For this review, take the finished solid that the model builds, in its own axes (mm). A direction names the side the tool comes from. Give positions to 0.01 mm unless a question says otherwise; leave off trailing zeros. Write each loop counter-clockwise with the first axis right and the second up, starting at its lowest first coordinate (ties: lowest second). Pieces come first, ordered by that corner, then holes.
1) For P1, Ø1.5, axis at y = 68, z = 1.5, coming from the -X side; P2, Ø1.5, axis at y = 65.5, z = 1.5, coming from the +X side; P3, Ø1.9, axis at x = 55.87, y = -64.6, coming from the +Z side; P4, Ø1, axis at x = -56.5, z = 1, coming from the +Y side, all flat-tipped, find the tip position at first contact; note any pin that passes through.
2) Wall thickness on line 1 along X through (y, z) = (19, 0.45); line 2 along Y through (x, z) = (-2.5, 1.2); line 3 along X through (y, z) = (44, 0.6): over which ranges is each line inside the solid? List them lowest first.
3) We need section C-C on z = 1.75. Give the number of separate pieces and of enclosed holes in the cut face, and give its area (3 significant figures).
4) Machinability: for faces 5 (the face through (68.796, -68.889, 1.479)), 6 (the face through (-51.49, 51.72, 1.48)), which of the approach directions +Z, -Z, +X, -X, +Y, -Y give a long, thin tool a straight path to every point of the face, cutting with its end or side? Answer none if there is none.
5) Draft analysis for pull direction Y (two halves, no side actions). For faces 1 (the face through (25.348, 85.358, 1.479)), 2 (the face through (38.828, 81.603, 1.479)), 3 (the face through (-68.889, -68.796, 1.479)), 4 (the face through (50.091, 50.293, 1.479)), state which applies: pulls with the +Y half, pulls with the -Y half, needs draft (parallel to the pull), parting line crosses it, or undercut.
6) We need section B-B on y = 9.5. Give the boundary of the cut face in (x, z).
7) We need section A-A on x = -5. Give the boundary of the cut face in (y, z).
from build123d import *

# Parameters (mm, degrees)
SKETCH2_R           = 1.6
SKETCH2_R_2         = 2.5
SKETCH2_W           = 82
SKETCH2_H           = 12.6
BOSS_EXTRUDE1_DEPTH = 3
FILLET2_R           = 1.5
FILLET3_R           = 3


with BuildPart() as part:
    # Sketch2 → Boss-Extrude1 (new body)
    # profile 1 of 2: a face of its own
    with BuildSketch(Plane.XY):
        with BuildLine():
            ThreePointArc((-65.540902989, 70.525765905), (-69.163190657, 68.495804286), (-70.6, 64.6))
            Line((-70.6, 64.6), (-70.6, -64.6))
            ThreePointArc((-70.6, -64.6), (-68.842640687, -68.842640687), (-64.6, -70.6))
            Line((-64.6, -70.6), (64.6, -70.6))
            ThreePointArc((64.6, -70.6), (68.842640687, -68.842640687), (70.6, -64.6))
            Line((70.6, -64.6), (70.6, 64.6))
            ThreePointArc((70.6, 64.6), (69.163190657, 68.495804286), (65.540902989, 70.525765905))
            ThreePointArc((65.540902989, 70.525765905), (64.340790015, 70.792848887), (63.182522555, 71.205184867))
            Line((63.182522555, 71.205184867), (13.781138102, 92.296857547))
            ThreePointArc((13.781138102, 92.296857547), (11.858510235, 92.897157125), (9.854586018, 93.1))
            Line((9.854586018, 93.1), (-9.854586018, 93.1))
            ThreePointArc((-9.854586018, 93.1), (-11.858510235, 92.897157125), (-13.781138102, 92.296857547))
            Line((-13.781138102, 92.296857547), (-63.182522555, 71.205184867))
            ThreePointArc((-63.182522555, 71.205184867), (-64.340790015, 70.792848887), (-65.540902989, 70.525765905))
        make_face()
        with Locations((-55.87, -64.6)):
            Circle(SKETCH2_R, mode=Mode.SUBTRACT)
        with Locations((-48.6, -64.6)):
            Circle(SKETCH2_R_2, mode=Mode.SUBTRACT)
        with BuildLine():
            Line((-11.9, 91.1), (-6, 91.1))
            Line((-6, 91.1), (6, 91.1))
            Line((6, 91.1), (11.9, 91.1))
            Line((11.9, 91.1), (41, 78.675901328))
            Line((41, 78.675901328), (41, 56))
            Line((41, 56), (-41, 56))
            ThreePointArc((-41, 56), (-51.606601718, 51.606601718), (-56, 41))
            Line((-56, 41), (-56, -41))
            ThreePointArc((-56, -41), (-55.457696912, -44.996873778), (-53.87, -48.704745291))
            Line((-53.87, -48.704745291), (-53.87, -61.6))
            Line((-53.87, -61.6), (-58.87, -61.6))
            Line((-58.87, -61.6), (-58.87, -68.6))
            Line((-58.87, -68.6), (-64.6, -68.6))
            ThreePointArc((-64.6, -68.6), (-67.428427125, -67.428427125), (-68.6, -64.6))
            Line((-68.6, -64.6), (-68.6, 64.6))
            ThreePointArc((-68.6, 64.6), (-67.428427125, 67.428427125), (-64.6, 68.6))
            Line((-64.6, 68.6), (-11.9, 91.1))
        make_face(mode=Mode.SUBTRACT)
        with Locations((0, -62.3)):
            Rectangle(SKETCH2_W, SKETCH2_H, mode=Mode.SUBTRACT)
        with Locations((48.6, -64.6)):
            Circle(SKETCH2_R_2, mode=Mode.SUBTRACT)
        with Locations((55.87, -64.6)):
            Circle(SKETCH2_R, mode=Mode.SUBTRACT)
        with BuildLine():
            Line((41, -54), (-41, -54))
            ThreePointArc((-41, -54), (-50.192388155, -50.192388155), (-54, -41))
            Line((-54, -41), (-54, 41))
            ThreePointArc((-54, 41), (-50.192388155, 50.192388155), (-41, 54))
            Line((-41, 54), (41, 54))
            ThreePointArc((41, 54), (50.192388155, 50.192388155), (54, 41))
            Line((54, 41), (54, -41))
            ThreePointArc((54, -41), (50.192388155, -50.192388155), (41, -54))
        make_face(mode=Mode.SUBTRACT)
        with BuildLine():
            Line((58.972044185, 61.502827435), (58.972044185, 71.002827435))
            Line((58.972044185, 71.002827435), (64.6, 68.6))
            ThreePointArc((64.6, 68.6), (67.428427125, 67.428427125), (68.6, 64.6))
            Line((68.6, 64.6), (68.6, -64.6))
            ThreePointArc((68.6, -64.6), (67.428427125, -67.428427125), (64.6, -68.6))
            Line((64.6, -68.6), (58.87, -68.6))
            Line((58.87, -68.6), (58.87, -61.6))
            Line((58.87, -61.6), (53.87, -61.6))
            Line((53.87, -61.6), (53.87, -48.704745291))
            ThreePointArc((53.87, -48.704745291), (55.457696912, -44.996873778), (56, -41))
            Line((56, -41), (56, 41))
            ThreePointArc((56, 41), (55.354105036, 45.354270159), (53.472044185, 49.333553495))
            Line((53.472044185, 49.333553495), (53.472044185, 61.502827435))
            Line((53.472044185, 61.502827435), (58.972044185, 61.502827435))
        make_face(mode=Mode.SUBTRACT)
        with Locations((48.6, 64.6)):
            Circle(SKETCH2_R_2, mode=Mode.SUBTRACT)
        with Locations((55.87, 64.6)):
            Circle(SKETCH2_R, mode=Mode.SUBTRACT)
    # profile 2 of 2: a face of its own
    with BuildSketch(Plane.XY):
        with BuildLine():
            ThreePointArc((-65.540902989, 70.525765905), (-69.163190657, 68.495804286), (-70.6, 64.6))
            Line((-70.6, 64.6), (-70.6, -64.6))
            ThreePointArc((-70.6, -64.6), (-68.842640687, -68.842640687), (-64.6, -70.6))
            Line((-64.6, -70.6), (64.6, -70.6))
            ThreePointArc((64.6, -70.6), (68.842640687, -68.842640687), (70.6, -64.6))
            Line((70.6, -64.6), (70.6, 64.6))
            ThreePointArc((70.6, 64.6), (69.163190657, 68.495804286), (65.540902989, 70.525765905))
            ThreePointArc((65.540902989, 70.525765905), (64.340790015, 70.792848887), (63.182522555, 71.205184867))
            Line((63.182522555, 71.205184867), (13.781138102, 92.296857547))
            ThreePointArc((13.781138102, 92.296857547), (11.858510235, 92.897157125), (9.854586018, 93.1))
            Line((9.854586018, 93.1), (-9.854586018, 93.1))
            ThreePointArc((-9.854586018, 93.1), (-11.858510235, 92.897157125), (-13.781138102, 92.296857547))
            Line((-13.781138102, 92.296857547), (-63.182522555, 71.205184867))
            ThreePointArc((-63.182522555, 71.205184867), (-64.340790015, 70.792848887), (-65.540902989, 70.525765905))
        make_face()
        with Locations((-55.87, -64.6)):
            Circle(SKETCH2_R, mode=Mode.SUBTRACT)
        with Locations((-48.6, -64.6)):
            Circle(SKETCH2_R_2, mode=Mode.SUBTRACT)
        with BuildLine():
            Line((-11.9, 91.1), (-6, 91.1))
            Line((-6, 91.1), (6, 91.1))
            Line((6, 91.1), (11.9, 91.1))
            Line((11.9, 91.1), (41, 78.675901328))
            Line((41, 78.675901328), (41, 56))
            Line((41, 56), (-41, 56))
            ThreePointArc((-41, 56), (-51.606601718, 51.606601718), (-56, 41))
            Line((-56, 41), (-56, -41))
            ThreePointArc((-56, -41), (-55.457696912, -44.996873778), (-53.87, -48.704745291))
            Line((-53.87, -48.704745291), (-53.87, -61.6))
            Line((-53.87, -61.6), (-58.87, -61.6))
            Line((-58.87, -61.6), (-58.87, -68.6))
            Line((-58.87, -68.6), (-64.6, -68.6))
            ThreePointArc((-64.6, -68.6), (-67.428427125, -67.428427125), (-68.6, -64.6))
            Line((-68.6, -64.6), (-68.6, 64.6))
            ThreePointArc((-68.6, 64.6), (-67.428427125, 67.428427125), (-64.6, 68.6))
            Line((-64.6, 68.6), (-11.9, 91.1))
        make_face(mode=Mode.SUBTRACT)
        with Locations((0, -62.3)):
            Rectangle(SKETCH2_W, SKETCH2_H, mode=Mode.SUBTRACT)
        with Locations((48.6, -64.6)):
            Circle(SKETCH2_R_2, mode=Mode.SUBTRACT)
        with Locations((55.87, -64.6)):
            Circle(SKETCH2_R, mode=Mode.SUBTRACT)
        with BuildLine():
            Line((41, -54), (-41, -54))
            ThreePointArc((-41, -54), (-50.192388155, -50.192388155), (-54, -41))
            Line((-54, -41), (-54, 41))
            ThreePointArc((-54, 41), (-50.192388155, 50.192388155), (-41, 54))
            Line((-41, 54), (41, 54))
            ThreePointArc((41, 54), (50.192388155, 50.192388155), (54, 41))
            Line((54, 41), (54, -41))
            ThreePointArc((54, -41), (50.192388155, -50.192388155), (41, -54))
        make_face(mode=Mode.SUBTRACT)
        with BuildLine():
            Line((58.972044185, 61.502827435), (58.972044185, 71.002827435))
            Line((58.972044185, 71.002827435), (64.6, 68.6))
            ThreePointArc((64.6, 68.6), (67.428427125, 67.428427125), (68.6, 64.6))
            Line((68.6, 64.6), (68.6, -64.6))
            ThreePointArc((68.6, -64.6), (67.428427125, -67.428427125), (64.6, -68.6))
            Line((64.6, -68.6), (58.87, -68.6))
            Line((58.87, -68.6), (58.87, -61.6))
            Line((58.87, -61.6), (53.87, -61.6))
            Line((53.87, -61.6), (53.87, -48.704745291))
            ThreePointArc((53.87, -48.704745291), (55.457696912, -44.996873778), (56, -41))
            Line((56, -41), (56, 41))
            ThreePointArc((56, 41), (55.354105036, 45.354270159), (53.472044185, 49.333553495))
            Line((53.472044185, 49.333553495), (53.472044185, 61.502827435))
            Line((53.472044185, 61.502827435), (58.972044185, 61.502827435))
        make_face(mode=Mode.SUBTRACT)
        with Locations((48.6, 64.6)):
            Circle(SKETCH2_R_2, mode=Mode.SUBTRACT)
        with Locations((55.87, 64.6)):
            Circle(SKETCH2_R, mode=Mode.SUBTRACT)
    extrude(amount=BOSS_EXTRUDE1_DEPTH)

    # Fillet2
    fillet2_edges = [part.edges().sort_by_distance(p)[0] for p in [
        (58.972044185, 71.002827435, 1.5),
        (58.972044185, 61.502827435, 1.5),
        (53.472044185, 61.502827435, 1.5),
        (53.472044185, 49.333553495, 1.5),
        (53.87, -48.704745291, 1.5),
        (53.87, -61.6, 1.5),
        (58.87, -61.6, 1.5),
        (58.87, -68.6, 1.5),
        (-58.87, -68.6, 1.5),
        (-58.87, -61.6, 1.5),
        (-53.87, -61.6, 1.5),
        (-53.87, -48.704745291, 1.5),
    ]]
    fillet(fillet2_edges, radius=FILLET2_R)

    # Fillet3
    fillet3_edges = [part.edges().sort_by_distance(p)[0] for p in [
        (-41, -68.6, 1.5),
        (41, -68.6, 1.5),
        (41, -56, 1.5),
        (-41, -56, 1.5),
        (41, 56, 1.5),
        (41, 78.675901328, 1.5),
    ]]
    fillet(fillet3_edges, radius=FILLET3_R)


solid = part.part
Results list:
1. P1: stops at x = -69.98
1. P2: stops at x = 70.6
1. P3: passes through
1. P4: stops at y = 74.27
2. line 1: x = -70.6 to -68.6, -56 to -54, 54 to 56, 68.6 to 70.6
2. line 2: y = -70.6 to -68.6, -56 to -54, 54 to 56, 91.1 to 93.1
2. line 3: x = -70.6 to -68.6, -55.7 to -53.65, 53.65 to 55.7, 68.6 to 70.6
3. separate pieces: 1
3. enclosed holes: 10
3. area: 2,640 mm2
4. face 5: +Z, -Z, +X, -Y
4. face 6: +Z, -Z
5. face 1: undercut
5. face 2: pulls with the +Y half
5. face 3: pulls with the -Y half
5. face 4: undercut
6. outline: (-70.6, 0) - (-68.6, 0) - (-68.6, 3) - (-70.6, 3) - close; (-56, 0) - (-54, 0) - (-54, 3) - (-56, 3) - close; (54, 0) - (56, 0) - (56, 3) - (54, 3) - close; (68.6, 0) - (70.6, 0) - (70.6, 3) - (68.6, 3) - close
7. outline: (-70.6, 0) - (-68.6, 0) - (-68.6, 3) - (-70.6, 3) - close; (-56, 0) - (-54, 0) - (-54, 3) - (-56, 3) - close; (54, 0) - (56, 0) - (56, 3) - (54, 3) - close; (91.1, 0) - (93.1, 0) - (93.1, 3) - (91.1, 3) - close
